```python
from build123d import *

# Parameters (mm, degrees)
SKETCH1_W           = 25.4
SKETCH1_H           = 25.4
BOSS_EXTRUDE1_DEPTH = 3
SKETCH2_W           = 3
SKETCH2_H           = 25.4
BOSS_EXTRUDE2_DEPTH = 17
SKETCH3_W           = 25.4
SKETCH3_H           = 2.5
BOSS_EXTRUDE3_DEPTH = 22.4
SKETCH4_W           = 2
SKETCH4_H           = 25.4
BOSS_EXTRUDE4_DEPTH = 10
CHAMFER1_SIZE       = 1.5
CHAMFER2_SIZE       = 3
CHAMFER3_SIZE       = 2
CHAMFER4_SIZE       = 1.5


with BuildPart() as part:
    # Sketch1 → Boss-Extrude1 (new body)
    with BuildSketch(Plane(origin=(0, 0, 0), x_dir=(1, 0, 0), z_dir=(0, 1, 0))):
        Rectangle(SKETCH1_W, SKETCH1_H)
    extrude(amount=BOSS_EXTRUDE1_DEPTH)

    # Sketch2 → Boss-Extrude2 (add)
    with BuildSketch(Plane(origin=(0, 3, 0), x_dir=(1, 0, 0), z_dir=(0, 1, 0))):
        with Locations((11.2, 0)):
            Rectangle(SKETCH2_W, SKETCH2_H)
    extrude(amount=BOSS_EXTRUDE2_DEPTH)

    # Sketch3 → Boss-Extrude3 (add)
    with BuildSketch(Plane.ZY.offset(-9.7)):
        with Locations((0, 18.75)):
            Rectangle(SKETCH3_W, SKETCH3_H)
    extrude(amount=BOSS_EXTRUDE3_DEPTH)

    # Sketch4 → Boss-Extrude4 (add)
    with BuildSketch(Plane.XZ.offset(-17.5)):
        with Locations((-11.7, 0)):
            Rectangle(SKETCH4_W, SKETCH4_H)
    extrude(amount=BOSS_EXTRUDE4_DEPTH)

    # Chamfer1
    chamfer1_edges = [part.edges().sort_by_distance(p)[0] for p in [
        (-12.7, 7.5, 0),
    ]]
    chamfer(chamfer1_edges, length=CHAMFER1_SIZE)

    # Chamfer2
    chamfer2_edges = [part.edges().sort_by_distance(p)[0] for p in [
        (12.7, 20, 0),
        (-12.7, 20, 0),
    ]]
    chamfer(chamfer2_edges, length=CHAMFER2_SIZE)

    # Chamfer3
    chamfer3_edges = [part.edges().sort_by_distance(p)[0] for p in [
        (9.7, 17.5, 0),
        (-10.7, 17.5, 0),
    ]]
    chamfer(chamfer3_edges, length=CHAMFER3_SIZE)

    # Chamfer4
    chamfer4_edges = [part.edges().sort_by_distance(p)[0] for p in [
        (-12.7, 3, 0),
    ]]
    chamfer(chamfer4_edges, length=CHAMFER4_SIZE)


solid = part.part
```
The listing builds one solid part. Answer for the finished solid, in the listing's coordinates (mm). A direction names the side the tool comes from. Coordinates: 2 decimals unless noted, no trailing zeros. Loops run counter-clockwise (first coordinate to the right, second up) from the corner with the lowest first, then second, coordinate; pieces in that order, holes last. Notation, with made-up numbers: (-12.75, 67.5) - (-4.75, 67.5) arc R10 ccw to (-4.75, 80.5) - close; hole circle Ø6 at (88.25, -26.5). An arc over 180 degrees is marked (long way). Use a Markdown table: item, result. Add a question column.
1) The part is cut by section C-C, the plane z = -5.25. Give the vertices of the cut face in (x, y), and give its area (3 significant figures).
2) Find the intervals of material crossed by line 1 (Y direction, x = -7.25, z = -8); line 2 (X direction, y = 9.5, z = 1); line 3 (Y direction, x = 8.5, z = 0.75), in increasing order.
3) For faces 1 (the flat face through (-1, 3, 0)), 2 (the flat face through (0, 0, 0)), 3 (the flat face through (-9.7, 16.5, -0.2)), determine the directions among +Z, -Z, +X, -X, +Y, -Y from which every point of the face is accessible in a straight line to the end or side of a thin tool.
4) The part is cut by section A-A, the plane x = 5.25. Give the vertices of the cut face in (y, z), and give its area (3 significant figures).
5) The mould has two halves that part along Y. Classify faces 4 (the flat face through (0, 17.5, 0)), 5 (the flat face through (12.7, 8, 0)), 6 (the flat face through (0, 20, 0)), 7 (the flat face through (-10.7, 12, 0)): released by +Y, released by -Y, zero draft, split by the parting line, or undercut.
6) The part is cut by section D-D, the plane x = 10.75. Give the vertices of the cut face in (y, z).
7) The part is cut by section B-B, the plane y = 14. Give the vertices of the cut face in (x, z), and give its area (3 significant figures).
Here are the results:
| question | item | result |
|---|---|---|
| 1 | outline | (-12.7, 0) - (12.7, 0) - (12.7, 17) - (9.7, 20) - (-9.7, 20) - (-12.7, 17) - (-12.7, 9) - (-11.2, 7.5) - (-10.7, 7.5) - (-10.7, 15.5) - (-8.7, 17.5) - (7.7, 17.5) - (9.7, 15.5) - (9.7, 3) - (-11.2, 3) - (-12.7, 1.5) - close |
| 1 | area | 196 mm^2 |
| 2 | line 1 | y = 0 to 3, 17.5 to 20 |
| 2 | line 2 | x = -12.7 to -10.7, 9.7 to 12.7 |
| 2 | line 3 | y = 0 to 3, 16.7 to 20 |
| 3 | face 1 | +Z, -Z, -X |
| 3 | face 2 | +Z, -Z, +X, -X, -Y |
| 3 | face 3 | +Z, -Z |
| 4 | outline | (0, -12.7) - (3, -12.7) - (3, 12.7) - (0, 12.7) - close; (17.5, -12.7) - (20, -12.7) - (20, 12.7) - (17.5, 12.7) - close |
| 4 | area | 140 mm^2 |
| 5 | face 4 | undercut |
| 5 | face 5 | zero draft |
| 5 | face 6 | released by +Y |
| 5 | face 7 | undercut |
| 6 | outline | (0, -12.7) - (18.95, -12.7) - (18.95, 12.7) - (0, 12.7) - close |
| 7 | outline | (-12.7, -12.7) - (-10.7, -12.7) - (-10.7, 12.7) - (-12.7, 12.7) - close; (9.7, -12.7) - (12.7, -12.7) - (12.7, 12.7) - (9.7, 12.7) - close |
| 7 | area | 127 mm^2 |
